from build123d import *

# Parameters (mm, degrees)
SKETCH1_W = 166.8859375
SKETCH1_H = 69.85
FILLET1_R = 9.525
SHELL1_T  = -4.7625


with BuildPart() as part:
    # Sketch1 → Revolve1 (revolve)
    with BuildSketch(Plane(origin=(0, 0, 0), x_dir=(0, 0, -1), z_dir=(1, 0, 0)), mode=Mode.PRIVATE) as revolve1_sk:
        with Locations((-83.44296875, 34.925)):
            Rectangle(SKETCH1_W, SKETCH1_H)
    revolve(revolve1_sk.sketch.rotate(Axis((0, 0, 0), (0, 1, 0)), 180), axis=Axis((0, 0, 0), (0, 1, 0)))

    # Fillet1
    fillet1_edges = [part.edges().sort_by_distance(p)[0] for p in [
        (0, 69.85, 166.8859375),
    ]]
    fillet(fillet1_edges, radius=FILLET1_R)

    # Shell1
    shell1_openings = [part.faces().sort_by_distance(p)[0] for p in [
        (0, 0, 0),
    ]]
    offset(amount=SHELL1_T, openings=shell1_openings, kind=Kind.INTERSECTION)


solid = part.part
Geometry check sheet. Reference: the model listing, model coordinates, mm. Coordinates: 2 decimals unless noted, no trailing zeros. Order: outer loops, then holes, each group sorted by start corner. A loop starts at its lowest first (then second) coordinate and runs counter-clockwise, first axis right, second up. Notation, with made-up numbers: (56.25, 68.5) - (92.25, 68.5) arc R26 ccw to (92.25, 94.5) - close; hole circle Ø2 at (57.5, -23.75). An arc over 180 degrees is marked (long way). One line per item, written item: value.
(1) Depth check by flat-ended pin: pin 1 Ø10 at (x, y) = (-27.5, 33) entering from +Z; pin 2 Ø10 at (x, y) = (112.5, 51) entering from +Z; pin 3 Ø4 at (x, y) = (-42.5, 30.5) entering from +Z. Enter the tip coordinate at first touch or a pass-through.
Data:
pin 1: stops at z = 165.36
pin 2: stops at z = 127.65
pin 3: stops at z = 161.9
(2) Release check for a two-part mould opening along Z. For faces 1 (the face through (-2, 65.087, 2)), 2 (the face through (-2, 69.85, 2)), 3 (the face through (-48.697, 30.585, -154.637)), 4 (the face through (162.917, 30.585, 36.178)) record: +Z half, -Z half, draft (parallel to the pull), parting line (faces both ways), or undercut.
Data:
face 1: undercut
face 2: draft
face 3: undercut
face 4: parting line
(3) Sectioned sample at B-B (y = 30). Enter the section's corners in (x, z).
Data:
outline: circle Ø333.77 at (0, 0); hole circle Ø324.25 at (0, 0)
(4) Thickness scan on probe 1 along X at (y, z) = (14, 0); probe 2 along Y at (x, z) = (-9.5, 65); probe 3 along X at (y, z) = (4, 44). Record the ranges inside material, lowest first. Write a range as from..to.
Data:
probe 1: x = -166.89..-162.12, 162.12..166.89
probe 2: y = 65.09..69.85
probe 3: x = -160.98..-156.04, 156.04..160.98
